The drawing under review shows one solid part. Ordinate dimensions are in mm from its lowest x, y, z. A direction names the side the tool comes from. Give positions to 0.01 mm unless a question says otherwise; leave off trailing zeros. Order: outer loops, then holes, each group sorted by start corner. A loop starts at its lowest first (then second) coordinate and runs counter-clockwise, first axis right, second up. Notation, with made-up numbers: (73, 20.5) - (82, 20.5) arc R17 cw to (82, 50.5) - close; hole circle Ø7 at (50, 67.5). An arc over 180 degrees is marked (long way). Use CSV: the item, a comma, the result in double quotes.
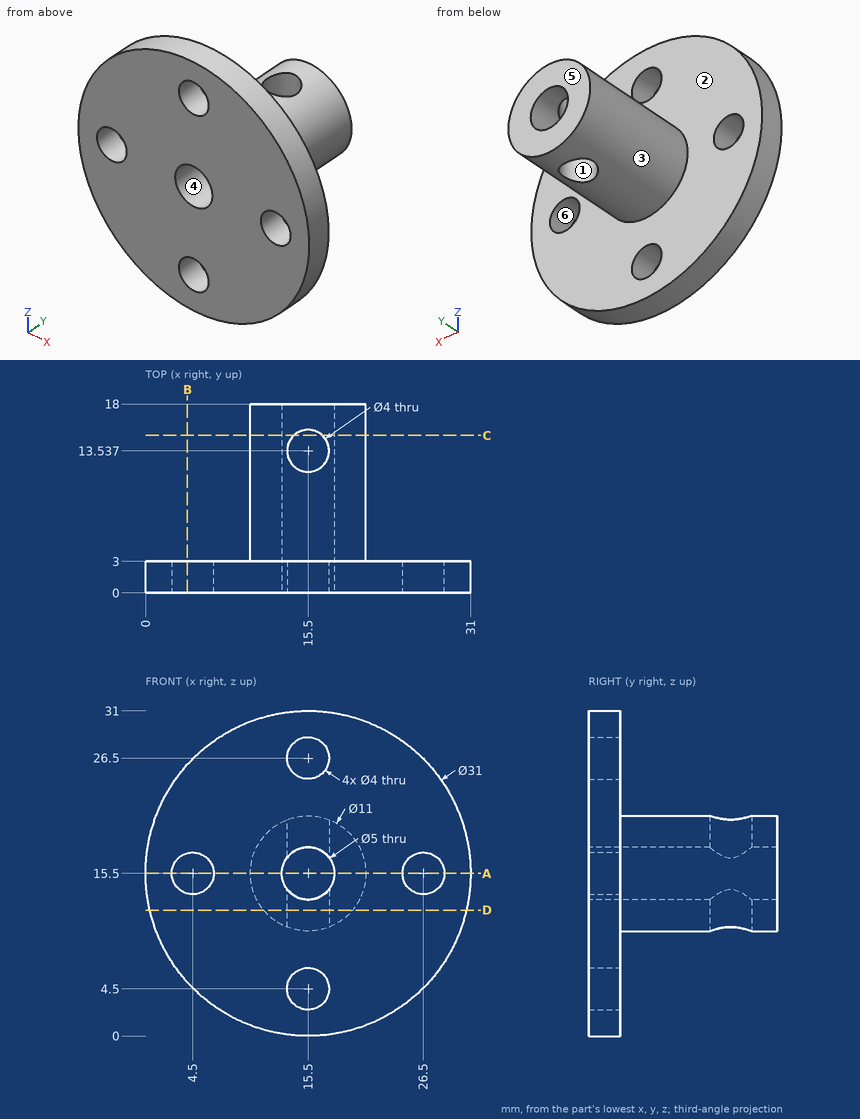
Item 1: Wall thickness on L1, parallel to Z at x = 15.5, y = 2.45; L2, parallel to X at y = 6.75, z = 15.5; L3, parallel to Y at x = 11, z = 19: over which ranges is each line inside the solid? List them lowest first.
Results list:
L1,"z = 0 to 2.5, 6.5 to 13, 18 to 24.5, 28.5 to 31"
L2,"x = 10 to 13, 18 to 21"
L3,"y = 0 to 3"
Item 2: Take a section at C-C, the plane y = 15. Give the boundary of the cut face in (x, z) (3 decimals).
Results list:
outline,"(14.136, 10.172) - (14.136, 13.405) arc R2.5 cw to (14.136, 17.595) - (14.136, 20.828) arc R5.5 ccw to start; (16.864, 10.172) arc R5.5 ccw to (16.864, 20.828) - (16.864, 17.595) arc R2.5 cw to (16.864, 13.405) - close"
Item 3: Tool access review of the marked faces 1 and 2: name each direction out of +Z, -Z, +X, -X, +Y, -Y from which nothing blocks a thin tool from reaching the whole face with its end or side.
Results list:
face 1,"+Z, -Z"
face 2,"+Y"
Item 4: Take a section at A-A, the plane z = 15.5. Give the boundary of the cut face in (x, y), and give its area (3 significant figures).
Results list:
outline,"(0, 0) - (2.5, 0) - (2.5, 3) - (0, 3) - close; (6.5, 0) - (13, 0) - (13, 18) - (10, 18) - (10, 3) - (6.5, 3) - close; (18, 0) - (24.5, 0) - (24.5, 3) - (21, 3) - (21, 18) - (18, 18) - close; (28.5, 0) - (31, 0) - (31, 3) - (28.5, 3) - close"
area,"144 mm2"
Item 5: Mouldability with a two-part tool opening along Z and no side actions: class the marked faces 3, 4, 5 and 6 as pulls with the +Z half, pulls with the -Z half, needs draft (parallel to the pull), parting line crosses it, or undercut.
Results list:
face 3,"parting line crosses it"
face 4,"undercut"
face 5,"needs draft"
face 6,"undercut"
Item 6: Clearance check with flat-ended pins moving along their axes: pin 1 (1 mm diameter, centred on x = 23, z = 15.5, fed in from +Y); pin 2 (10 mm diameter, centred on x = 5.5, y = 8.5, fed in from +Z); pin 3 (6.5 mm diameter, centred on x = 15.5, y = 13.54, fed in from +Z); pin 4 (4 mm diameter, centred on x = 15.5, z = 15.5, fed in from -Y). State where each tip first meets the part, or that it passes through.
Results list:
pin 1,"stops at y = 3"
pin 2,"stops at z = 17.79"
pin 3,"stops at z = 21"
pin 4,"passes through"
Item 7: Take a section at D-D, the plane z = 12. Give the boundary of the cut face in (x, y), and give its area (3 significant figures).
Results list:
outline,"(0.4, 0) - (30.6, 0) - (30.6, 3) - (19.74, 3) - (19.74, 18) - (11.26, 18) - (11.26, 3) - (0.4, 3) - close; hole circle Ø4 at (15.5, 13.54)"
area,"205 mm2"
Item 8: Take a section at B-B, the plane x = 4. Give the boundary of the cut face in (y, z).
Results list:
outline,"(0, 5.11) - (3, 5.11) - (3, 13.56) - (0, 13.56) - close; (0, 17.44) - (3, 17.44) - (3, 25.89) - (0, 25.89) - close"
